Solid Edge part; units mm, degrees
sketch "Sketch1" plane through (0, 0, 0) normal (0, 0, 1) x (1, 0, 0)
  circle A0 centre (0, 0) radius 2.75
extrude "Protrusion1" add sketch "Sketch1" along normal blind 3
sketch "Sketch2" plane through (0, 0, 3) normal (0, 0, 1) x (0, 1, 0)
  line L0 (0, 1.4434) -> (1.25, 0.7217)
  line L1 (1.25, 0.7217) -> (1.25, -0.7217)
  line L2 (1.25, -0.7217) -> (0, -1.4434)
  line L3 (0, -1.4434) -> (-1.25, -0.7217)
  line L4 (-1.25, -0.7217) -> (-1.25, 0.7217)
  line L5 (-1.25, 0.7217) -> (0, 1.4434)
extrude "Cutout1" cut sketch "Sketch2" against normal blind 1.3
fillet "Round1" radius 0.3 1 edges at (-2.75, 0, 3)
sketch "Sketch3" plane through (0, 0, 0) normal (1, 0, 0) x (0, 1, 0)
  line L0 (-1.1935, -12) -> (0, -12)
  line L1 (-1.5, -11.6935) -> (-1.1935, -12)
  line L2 (-1.5, -1.5) -> (-1.5, -11.6935)
  line L3 (-1.1935, -1.5) -> (-1.5, -1.5)
  line L4 (-1.1935, -1.49) -> (-1.1935, -1.5)
  line L5 (-1.5, -1.49) -> (-1.1935, -1.49)
  line L6 (-1.5, -0.1) -> (-1.5, -1.49)
  arc A0 (-1.5, -0.1) -> (-1.6, 0) centre (-1.6, -0.1) ccw
revolve "RevolvedProtrusion1" add sketch "Sketch3" angle 360 about axis through (0, 0, -60.325) along (0, 0, 1) material side at (0, -0.5968, -11.95)
cosmetic_thread "Thread1"
sketch "Sketch4" plane through (0, 0, 0) normal (0, -1, 0) x (1, 0, 0)
  line L0 (-1.435, 3) -> (0, 2.1715)
revolve "RevolvedCutout1" cut sketch "Sketch4" angle 360 about axis through (0, 0, 57.15) along (0, 0, -1) material side at (-0.6925, 0, 2.6291)
properties material "Steel"
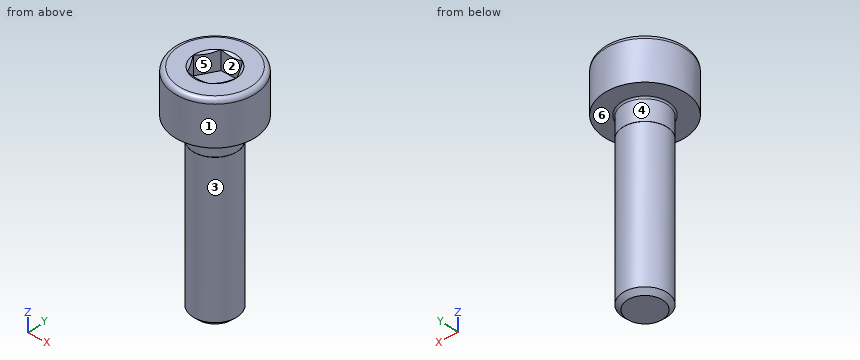
Verification items for the finished model (mm, model axes). Face numbers are marked on the shaded views. A direction names the side the tool comes from. Coordinates: 2 decimals unless noted, no trailing zeros. Order: outer loops, then holes, each group sorted by start corner. A loop starts at its lowest first (then second) coordinate and runs counter-clockwise, first axis right, second up.
Item 1: Depth check by flat-ended pin: pin 1 (1 mm diameter, centred on x = -1.5, y = 1.5, fed in from -Z); pin 2 (1 mm diameter, centred on x = -0.5, z = -7, fed in from -Y); pin 3 (1.5 mm diameter, centred on x = 1, z = 1.5, fed in from -Y). Enter the tip coordinate at first touch or a pass-through.
Filled in:
pin 1: stops at z = 0
pin 2: stops at y = -1.5
pin 3: stops at y = -2.74
Item 2: Section check C-C, the plane z = -8.5. Enter the section's corners in (x, y), then the cut area to 3 significant figures.
Filled in:
outline: circle Ø3 at (0, 0)
area: 7.07 mm2
Item 3: Section check B-B, the plane z = 0.5. Enter the section's corners in (x, y).
Filled in:
outline: circle Ø5.5 at (0, 0)
Item 4: Access from +Z, -Z, +X, -X, +Y, -Y to the whole of each face (thin tool, end or side, straight path). Record for the marked faces 1, 2 and 3.
Filled in:
face 1: +Z, -Z
face 2: +Z
face 3: -Z
Item 5: Material ranges on L1, parallel to X at y = 0.85, z = -6.75; L2, parallel to Y at x = -0.45, z = -7.25; L3, parallel to Z at x = 2.3, y = 0.15, recorded low to high.
Filled in:
L1: x = -1.24 to 1.24
L2: y = -1.43 to 1.43
L3: z = 0 to 3
Item 6: Release check for a two-part mould opening along X. For the marked faces 4, 5 and 6 record: +X half, -X half, draft (parallel to the pull), parting line (faces both ways), or undercut.
Filled in:
face 4: parting line
face 5: undercut
face 6: draft
